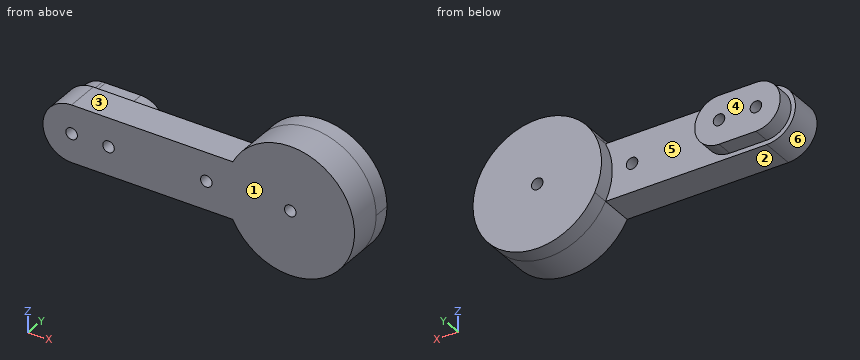
```python
from build123d import *

# Parameters (mm, degrees)
SKETCH1_R           = 0.625
BOSS_EXTRUDE1_DEPTH = 3.6
SKETCH2_R           = 0.625
BOSS_EXTRUDE2_DEPTH = 1.8


with BuildPart() as part:
    # Sketch1 → Boss-Extrude1 (new body)
    with BuildSketch(Plane(origin=(0, 0, 0), x_dir=(1, 0, 0), z_dir=(0, 1, 0))):
        with BuildLine():
            Line((-23.7, 3.107973286), (-6.230065085, 3.107973286))
            ThreePointArc((-6.230065085, 3.107973286), (6.962270385, 0), (-6.230065085, -3.107973286))
            Line((-6.230065085, -3.107973286), (-23.7, -3.107973286))
            ThreePointArc((-23.7, -3.107973286), (-26.807973286, 0), (-23.7, 3.107973286))
        make_face()
        with Locations((-23.7, 0)):
            Circle(SKETCH1_R, mode=Mode.SUBTRACT)
        with Locations((-19.7, 0)):
            Circle(SKETCH1_R, mode=Mode.SUBTRACT)
        with Locations((-9.1, 0)):
            Circle(SKETCH1_R, mode=Mode.SUBTRACT)
        Circle(SKETCH1_R, mode=Mode.SUBTRACT)
    extrude(amount=BOSS_EXTRUDE1_DEPTH)

    # Sketch2 → Boss-Extrude2 (add)
    with BuildSketch(Plane(origin=(0, 3.6, 0), x_dir=(1, 0, 0), z_dir=(0, 1, 0))):
        with BuildLine():
            ThreePointArc((-19.7, -2.633766086), (-17.066233914, 0), (-19.7, 2.633766086))
            Line((-19.7, 2.633766086), (-23.7, 2.633766086))
            ThreePointArc((-23.7, 2.633766086), (-26.332441924, 0.083506378), (-23.866928789, -2.628470768))
            Line((-23.866928789, -2.628470768), (-23.539752243, -2.628886543))
            Line((-23.539752243, -2.628886543), (-19.706693951, -2.63375758))
            Line((-19.706693951, -2.63375758), (-19.7, -2.633766086))
        make_face()
        with Locations((-19.7, 0)):
            Circle(SKETCH2_R, mode=Mode.SUBTRACT)
        with Locations((-23.7, 0)):
            Circle(SKETCH2_R, mode=Mode.SUBTRACT)
        with BuildLine():
            ThreePointArc((-6.230065085, -3.107973286), (1.596529247, -6.776747249), (6.962270385, 0))
            ThreePointArc((6.962270385, 0), (1.596529247, 6.776747249), (-6.230065085, 3.107973286))
            ThreePointArc((-6.230065085, 3.107973286), (-6.962270385, 0), (-6.230065085, -3.107973286))
        make_face()
        Circle(SKETCH2_R, mode=Mode.SUBTRACT)
    extrude(amount=BOSS_EXTRUDE2_DEPTH)


solid = part.part
```
Source: CAD feature listing. Evaluate the final solid. Frame: model axes, mm. Face numbers are marked on the shaded views. A direction names the side the tool comes from. Coordinates: 2 decimals unless noted, no trailing zeros. Order: outer loops, then holes, each group sorted by start corner. A loop starts at its lowest first (then second) coordinate and runs counter-clockwise, first axis right, second up. Notation, with made-up numbers: M 73.25,82 L 106.25,82 A16 cw 106.25,90 Z; hole C -37.75,-1 d9. An arc over 180 degrees is marked long. Write each question's results on one line, items separated by ' | '. Start each with the question number.
1) Section query B-B (y = 4.9). Return the cut outline in (x, z) (3 decimals), plus the area to 3 significant figures.
2) Draft query along X for the marked faces 4, 5 and 6. Return one class per face: released by +X, released by -X, zero draft, split by the parting line, or undercut.
3) Section query D-D (z = 4). Return the cut outline in (x, y), plus the area to 3 significant figures.
4) Section query A-A (x = 0). Return the cut outline in (y, z) (3 decimals).
5) Section query C-C (y = 1.5). Return the cut outline in (x, z) (3 decimals).
6) Contact query for flat-ended pins moving along their axis: pin 1 Ø1 at (x, z) = (-23.7, 0) entering from -Y; pin 2 Ø0.5 at (x, y) = (-21.5, 4.5) entering from -Z; pin 3 Ø3 at (x, y) = (-13.5, 2) entering from +Z; pin 4 Ø2 at (y, z) = (2, 5) entering from -X. Output: stop coordinate, or through.
7) Access query for the marked faces 1, 2 and 3. Directions: +Z, -Z, +X, -X, +Y, -Y. A direction counts if a zero-diameter tool reaches every point of the face in a straight line with its end or side. Return the directions, or none.
8) Line query: line 1 (X direction, y = 2, z = 0) (3 decimals); line 2 (Z direction, x = 0, y = 1.55) (3 decimals); line 3 (Z direction, x = -23.7, y = 3.1) (3 decimals). Output: solid intervals per line, ascending. Write a range as from..to.
Answers:
1) outline: M -23.867,2.628 A2.634 ccw -23.7,-2.634 L -19.7,-2.634 A2.634 ccw -19.7,2.634 Z; C 0,0 d13.925; hole C -23.7,0 d1.25; hole C -19.7,0 d1.25; hole C 0,0 d1.25 | area: 191 mm^2
2) face 4: zero draft | face 5: undercut | face 6: released by -X
3) outline: M -5.7,0 L 5.7,0 L 5.7,5.4 L -5.7,5.4 Z | area: 61.5 mm^2
4) outline: M 0,-6.962 L 5.4,-6.962 L 5.4,-0.625 L 0,-0.625 Z; M 0,0.625 L 5.4,0.625 L 5.4,6.962 L 0,6.962 Z
5) outline: M -23.7,-3.108 L -6.23,-3.108 A6.962 ccw long -6.23,3.108 L -23.7,3.108 A3.108 ccw Z; hole C -23.7,0 d1.25; hole C -19.7,0 d1.25; hole C -9.1,0 d1.25; hole C 0,0 d1.25
6) pin 1: passes through | pin 2: stops at z = -2.63 | pin 3: stops at z = 3.11 | pin 4: stops at x = -5.7
7) face 1: +Z, -Z, +X, -X, -Y | face 2: -Z, -X, +Y, -Y | face 3: +Z, -X, +Y, -Y
8) line 1: x = -26.808..-24.325, -23.075..-20.325, -19.075..-9.725, -8.475..-0.625, 0.625..6.962 | line 2: z = -6.962..-0.625, 0.625..6.962 | line 3: z = -3.108..-0.625, 0.625..3.108
